from build123d import *

# Parameters (mm, degrees)
DODANIE_WYCI_GNI_CIE2_DEPTH      = 10
DODANIE_WYCI_GNI_CIE3_DEPTH      = 5
DODANIE_WYCI_GNI_CIE4_DEPTH      = 2
DODANIE_WYCI_GNI_CIE4_DEPTH_BACK = 3
SFAZOWANIE2_SIZE                 = 1
ZAOKR_GLENIE2_R                  = 1
SZKIC5_W                         = 78
SZKIC5_H                         = 47.399243566
WYTNIJ_WYCI_GNI_CIE1_DEPTH       = 10


with BuildPart() as part:
    # Szkic1 → Dodanie-wyciągnięcie2 (new body)
    with BuildSketch(Plane(origin=(0, 0, 0), x_dir=(1, 0, 0), z_dir=(0, 1, 0))):
        with BuildLine():
            ThreePointArc((-35.198290521, 18.220532858), (0, 23.195615958), (35.198290521, 18.220532858))
            ThreePointArc((35.198290521, 18.220532858), (36.828860435, 17.052239434), (37.358722234, 15.117578161))
            ThreePointArc((37.358722234, 15.117578161), (34.64818175, -0.440013395), (28.93215854, -15.161180582))
            ThreePointArc((28.93215854, -15.161180582), (27.37301165, -16.588880533), (25.259425897, -16.633840931))
            ThreePointArc((25.259425897, -16.633840931), (0, -12.31341545), (-25.259425897, -16.633840931))
            ThreePointArc((-25.259425897, -16.633840931), (-27.37301165, -16.588880533), (-28.93215854, -15.161180582))
            ThreePointArc((-28.93215854, -15.161180582), (-34.64818175, -0.440013395), (-37.358722234, 15.117578161))
            ThreePointArc((-37.358722234, 15.117578161), (-36.828860435, 17.052239434), (-35.198290521, 18.220532858))
        make_face()
    extrude(amount=DODANIE_WYCI_GNI_CIE2_DEPTH)

    # Szkic3 → Dodanie-wyciągnięcie3 (add)
    with BuildSketch(Plane(origin=(0, 10, 0), x_dir=(1, 0, 0), z_dir=(0, 1, 0))):
        with BuildLine():
            ThreePointArc((-35.475442415, 19.181358975), (-37.649535634, 17.62363441), (-38.356018032, 15.044086045))
            ThreePointArc((-38.356018032, 15.044086045), (-35.611569929, -0.708123852), (-29.824041887, -15.613446096))
            ThreePointArc((-29.824041887, -15.613446096), (-27.745179368, -17.51704603), (-24.92706503, -17.576993227))
            ThreePointArc((-24.92706503, -17.576993227), (0, -13.31341545), (24.92706503, -17.576993227))
            ThreePointArc((24.92706503, -17.576993227), (27.745179368, -17.51704603), (29.824041887, -15.613446096))
            ThreePointArc((29.824041887, -15.613446096), (35.611569929, -0.708123852), (38.356018032, 15.044086045))
            ThreePointArc((38.356018032, 15.044086045), (37.649535634, 17.62363441), (35.475442415, 19.181358975))
            ThreePointArc((35.475442415, 19.181358975), (0, 24.195615958), (-35.475442415, 19.181358975))
        make_face()
    extrude(amount=DODANIE_WYCI_GNI_CIE3_DEPTH)

    # Szkic4 → Dodanie-wyciągnięcie4 (add, two sides: drawn at the far end of the back side and taken through both)
    with BuildSketch(Plane(origin=(0, 15, 0), x_dir=(1, 0, 0), z_dir=(0, 1, 0)).offset(-DODANIE_WYCI_GNI_CIE4_DEPTH_BACK)):
        with BuildLine():
            Line((-34.353845871, -4.804384042), (-38.327790803, -4.804384042))
            Line((-38.327790803, -4.804384042), (-42.5, -4.804384042))
            Line((-42.5, -4.804384042), (-47.5, -1.804384042))
            Line((-47.5, -1.804384042), (-47.5, 7.195615958))
            ThreePointArc((-47.5, 7.195615958), (-47.207106781, 7.90272274), (-46.5, 8.195615958))
            Line((-46.5, 8.195615958), (-37.556869269, 8.195615958))
            ThreePointArc((-37.556869269, 8.195615958), (-36.224623376, 1.629272522), (-34.353845871, -4.804384042))
        make_face()
        with BuildLine():
            Line((42.5, -4.804384042), (47.5, -1.804384042))
            Line((47.5, -1.804384042), (47.5, 7.195615958))
            ThreePointArc((47.5, 7.195615958), (47.207106781, 7.90272274), (46.5, 8.195615958))
            Line((46.5, 8.195615958), (37.556869269, 8.195615958))
            ThreePointArc((37.556869269, 8.195615958), (36.224623376, 1.629272522), (34.353845871, -4.804384042))
            Line((34.353845871, -4.804384042), (38.327790803, -4.804384042))
            Line((38.327790803, -4.804384042), (42.5, -4.804384042))
        make_face()
    extrude(amount=DODANIE_WYCI_GNI_CIE4_DEPTH + DODANIE_WYCI_GNI_CIE4_DEPTH_BACK)

    # Sfazowanie2
    sfazowanie2_edges = [part.edges().sort_by_distance(p)[0] for p in [
        (0, 15, -24.195615958),
        (-37.649535634, 15, -17.62363441),
        (-38.029401728, 15, -11.611337515),
        (-27.745179368, 15, 17.51704603),
        (0, 15, 13.31341545),
        (27.745179368, 15, 17.51704603),
        (32.284843088, 15, 10.291011463),
        (37.649535634, 15, -17.62363441),
        (38.029401728, 15, -11.611337515),
        (-32.284843088, 15, 10.291011463),
    ]]
    chamfer(sfazowanie2_edges, length=SFAZOWANIE2_SIZE)

    # Zaokrąglenie2
    zaokr_glenie2_edges = [part.edges().sort_by_distance(p)[0] for p in [
        (-36.224623376, 12, -1.629272522),
        (-36.224623376, 15, -1.629272522),
        (-38.426922936, 17, 4.804384042),
        (-45, 17, 3.304384042),
        (-47.5, 17, -2.695615958),
        (-42.028434635, 17, -8.195615958),
        (42.028434635, 17, -8.195615958),
        (47.5, 17, -2.695615958),
        (45, 17, 3.304384042),
        (38.426922936, 17, 4.804384042),
        (36.224623376, 12, -1.629272522),
        (36.224623376, 15, -1.629272522),
        (36.224623376, 17, -1.629272522),
    ]]
    fillet(zaokr_glenie2_edges, radius=ZAOKR_GLENIE2_R - 0.0001)  # a hair under: the kernel refuses the full size

    # Szkic5 → Wytnij-wyciągnięcie1 (cut)
    with BuildSketch(Plane(origin=(0, 15, 0), x_dir=(1, 0, 0), z_dir=(0, 1, 0))):
        with Locations((0, -5.950048289)):
            Rectangle(SZKIC5_W, SZKIC5_H)
    extrude(amount=WYTNIJ_WYCI_GNI_CIE1_DEPTH, mode=Mode.SUBTRACT)


solid = part.part
Here's how the part is built. I have some questions about the finished solid (model axes, mm). A direction names the side the tool comes from. Coordinates: 2 decimals unless noted, no trailing zeros. Order: outer loops, then holes, each group sorted by start corner. A loop starts at its lowest first (then second) coordinate and runs counter-clockwise, first axis right, second up.
Item 1: If we mould it in two halves opening along Z, with no side actions, what happens to faces 6 (the face through (35.551, 10.639, 0.924)), 7 (the face through (-0.356, 11.972, 13.314)), 8 (the face through (-0.499, 4.93, -23.195)), 9 (the face through (0, 10, -24))? For each: +Z half, -Z half, draft (parallel to the pull), parting line (faces both ways), or undercut.
Result sheet:
face 6: undercut
face 7: +Z half
face 8: -Z half
face 9: draft
Item 2: If we section it at A-A on y = 6.5: List the corners of the cut face in (x, z) for me.
Result sheet:
outline: (-37.36, -15.12) arc R3 ccw to (-35.2, -18.22) arc R127 ccw to (35.2, -18.22) arc R3 ccw to (37.36, -15.12) arc R79.94 ccw to (28.93, 15.16) arc R3 ccw to (25.26, 16.63) arc R76 cw to (-25.26, 16.63) arc R3 ccw to (-28.93, 15.16) arc R79.94 ccw to start
Item 3: For P1, Ø5, axis at x = -4, z = -1, coming from the +Y side; P2, Ø2.5, axis at x = -37.5, y = 14.5, coming from the +Z side; P3, Ø2.5, axis at x = 40, y = 12.5, coming from the -Z side, each with a flat end and sliding along its axis, tell me the tip position at first contact or that it passes through.
Result sheet:
P1: stops at y = 15
P2: stops at z = 4.8
P3: stops at z = -8.2
Item 4: I need wall thicknesses on line 1 (Y direction, x = -23, z = 5.5); line 2 (Y direction, x = 38, z = 0.5); line 3 (X direction, y = 13.25, z = -15.5). Which ranges of each line are inside material? Lowest first, please.
Result sheet:
line 1: y = 0 to 15
line 2: y = 12 to 15
line 3: x = -38.36 to 38.36
Item 5: If we section it at B-B on x = 40.5: List the corners of the cut face in (y, z) for me, plus the area to 3 significant figures.
Result sheet:
outline: (12, -8.2) - (16, -8.2) arc R1 ccw to (17, -7.2) - (17, 3.8) arc R1 ccw to (16, 4.8) - (12, 4.8) - close
area: 64.6 mm2
Item 6: For faces 1 (the face through (-43, 17, -2)), 2 (the face through (-44.96, 13.97, 3.33)), 3 (the face through (-27.34, 4.93, 16.6)), 4 (the face through (34.707, 4.93, 0.227)), 5 (the face through (-39, 16, -2)), which set-ups out of +Z, -Z, +X, -X, +Y, -Y let a thin tool reach every point of the face, with its end or its side?
Result sheet:
face 1: +Z, -Z, +X, -X, +Y
face 2: +Z, -X, +Y, -Y
face 3: +Z, -Y
face 4: +Z, +X, -Y
face 5: +Z, -Z, +Y
